Part model, mm, in its own coordinate system. Face numbers are marked on the shaded views. A direction names the side the tool comes from. Round coordinates to 2 decimals unless told otherwise and drop trailing zeros. Loops run counter-clockwise (first coordinate to the right, second up) from the corner with the lowest first, then second, coordinate; pieces in that order, holes last.
1) Band-saw the part on A-A, the plane y = 16. Write the cut outline in (x, z), then the cut area to 3 significant figures.
2) Probe line 1 (Z direction, x = 11.5, y = 19); line 2 (X direction, y = 22, z = 46.5); line 3 (Y direction, x = 7, z = 14.5). List the from-to ranges inside material, lowest first.
3) 3-axis set-ups, long thin cutter, end or side, ignore diameter. For the marked faces 1, 2, 3 and 4: which of +Z, -Z, +X, -X, +Y, -Y reach the whole face in a straight line?
4) Band-saw the part on C-C, the plane x = -4. Write the cut outline in (y, z).
5) Band-saw the part on B-B, the plane z = 23. Write the cut outline in (x, y), then the cut area to 3 significant figures.
6) Band-saw the part on D-D, the plane y = 26.5. Write the cut outline in (x, z), then the cut area to 3 significant figures.
7) Drop flat-ended pins along their axis: P1, Ø5, axis at y = 37, z = 30, coming from the -X side; P2, Ø3, axis at x = -11.5, y = 27.5, coming from the +Z side; P3, Ø5, axis at y = 18.5, z = 36.5, coming from the -X side; P4, Ø1.5, axis at y = 18, z = 53, coming from the +X side. Give the stop position or say it passes through.
from build123d import *

# Parameters (mm, degrees)
SALIENTE_EXTRUIR1_DEPTH = 15.5
CROQUIS2_W              = 13
CROQUIS2_H              = 7
SALIENTE_EXTRUIR2_DEPTH = 42
NERVIO1_REACH           = 90.206
CROQUIS3_WALL_W         = 240.185231722
CROQUIS3_WALL_H         = 10


with BuildPart() as part:
    # Croquis1 → Saliente-Extruir1 (new, symmetric)
    with BuildSketch(Plane(origin=(0, 0, 0), x_dir=(0, 0, -1), z_dir=(1, 0, 0))):
        Polygon((0, 0), (-76, 0), (-76, 12), (-14, 12), (-14, 42), (0, 42), align=None)
    extrude(amount=SALIENTE_EXTRUIR1_DEPTH, both=True)

    # Croquis2 → Saliente-Extruir2 (add)
    with BuildSketch(Plane(origin=(0, 42, 0), x_dir=(1, 0, 0), z_dir=(0, 1, 0))):
        with Locations((0, 3.5)):
            Rectangle(CROQUIS2_W, CROQUIS2_H)
    extrude(amount=-SALIENTE_EXTRUIR2_DEPTH)

    # Croquis3 wall → Nervio1 (add, up to next)
    with BuildSketch(Plane(origin=(0, 27, 41), x_dir=(0, 0.485642931179, -0.874157276122), z_dir=(0, 0.874157276122, 0.485642931179)), mode=Mode.PRIVATE) as nervio1_sk1:
        Rectangle(CROQUIS3_WALL_W, CROQUIS3_WALL_H)
    nervio1_tool1 = extrude(nervio1_sk1.sketch, amount=-NERVIO1_REACH, mode=Mode.PRIVATE) - part.part
    add(nervio1_tool1.solids().sort_by_distance((0, 27, 41))[0])


solid = part.part
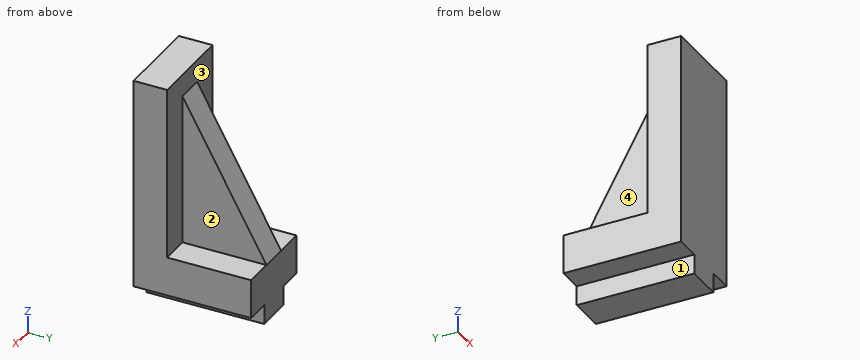
Reported:
1. outline: (-15.5, 0) - (-6.5, 0) - (-6.5, -7) - (6.5, -7) - (6.5, 0) - (15.5, 0) - (15.5, 14) - (5, 14) - (5, 60.8) - (-5, 60.8) - (-5, 14) - (-15.5, 14) - close
1. area: 993 mm2
2. line 1: z = 0 to 14
2. line 2: x = -5 to 5
2. line 3: y = 0 to 12
3. face 1: -Z, -X, +Y, -Y
3. face 2: +Z, +X, +Y
3. face 3: +Z, +Y
3. face 4: +Z, -X, +Y
4. outline: (0, -7) - (42, -7) - (42, 14) - (12, 68) - (12, 76) - (0, 76) - close
5. outline: (-15.5, 0) - (15.5, 0) - (15.5, 12) - (5, 12) - (5, 37) - (-5, 37) - (-5, 12) - (-15.5, 12) - close
5. area: 622 mm2
6. outline: (-15.5, 0) - (-6.5, 0) - (-6.5, -7) - (6.5, -7) - (6.5, 0) - (15.5, 0) - (15.5, 14) - (5, 14) - (5, 41.9) - (-5, 41.9) - (-5, 14) - (-15.5, 14) - close
6. area: 804 mm2
7. P1: passes through
7. P2: stops at z = 14
7. P3: stops at x = -5
7. P4: stops at x = 5
